Study the drawing (mm; zero at the part's minimum x, y, z) and answer. Round coordinates to 2 decimals unless told otherwise and drop trailing zeros. Order: outer loops, then holes, each group sorted by start corner. A loop starts at its lowest first (then second) coordinate and runs counter-clockwise, first axis right, second up. Notation, with made-up numbers: (-10.5, -26) - (46.5, -26) arc R28 cw to (46.5, 13) - close; hole circle Ø4 at (81, 52). An arc over 180 degrees is marked (long way). Put each result on its own line as item: value. Start each with the question number.
Q1. Section A-A on y = 116 is taken. Give the vertices of the cut face in (x, z), then the cut area to 3 significant figures.
Q2. Find the intervals of material crossed by line 1 along Y through (x, z) = (286, 11.75); line 2 along Z through (x, y) = (300, 14); line 3 along X through (y, z) = (106, 22.5), in increasing order. Write a range as from..to.
Q3. Section C-C on z = 12.5 is taken. Give the vertices of the cut face in (x, y).
Q4. Section B-B on x = 269 is taken. Give the vertices of the cut face in (y, z).
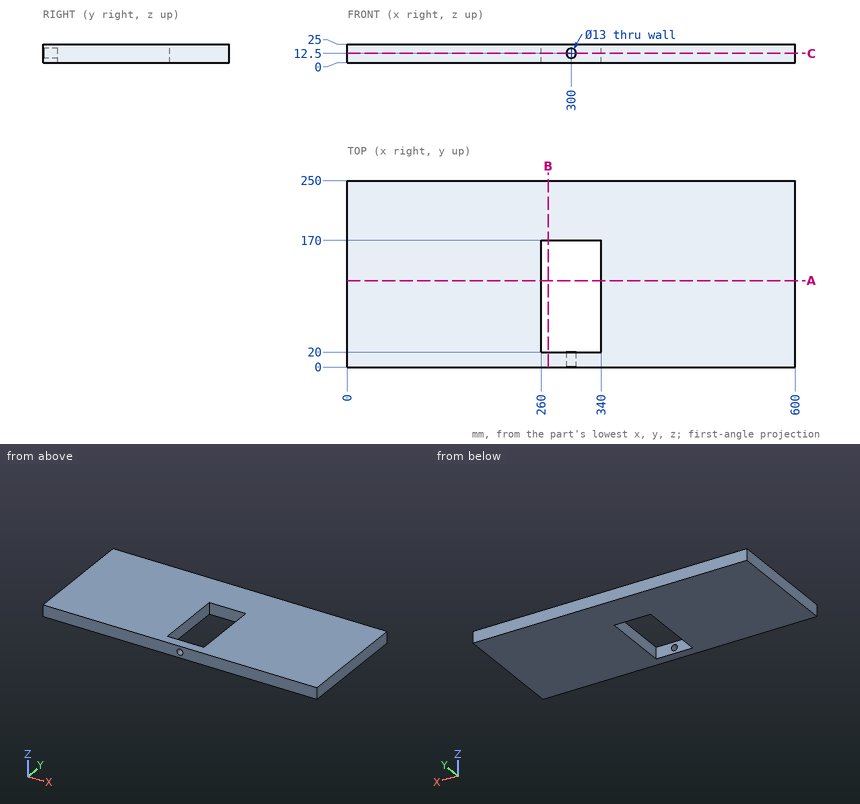
Findings:
1. outline: (0, 0) - (260, 0) - (260, 25) - (0, 25) - close; (340, 0) - (600, 0) - (600, 25) - (340, 25) - close
1. area: 13,000 mm2
2. line 1: 0..20, 170..250
2. line 2: 0..6, 19..25
2. line 3: 0..260, 340..600
3. outline: (0, 0) - (293.5, 0) - (293.5, 20) - (260, 20) - (260, 170) - (340, 170) - (340, 20) - (306.5, 20) - (306.5, 0) - (600, 0) - (600, 250) - (0, 250) - close
4. outline: (0, 0) - (20, 0) - (20, 25) - (0, 25) - close; (170, 0) - (250, 0) - (250, 25) - (170, 25) - close
